Autodesk Inventor part; units mm, degrees
ref_plane "YZ Plane" through (0, 0, 0) normal (1, 0, 0) x (0, 1, 0)
ref_plane "XZ Plane" through (0, 0, 0) normal (0, 1, 0) x (-1, 0, 0)
ref_plane "XY Plane" through (0, 0, 0) normal (0, 0, 1) x (1, 0, 0)
sketch "Sketch1" plane through (0, 0, 0) normal (0, 1, 0) x (-1, 0, 0)
  circle A0 centre (0, 0) radius 1.4
  dimension "d0" = 2.8
extrude "Extrusion1" add sketch "Sketch1" along normal blind 5.5
sketch "Sketch2" plane through (0, 5.5, 0) normal (0, 1, 0) x (1, 0, 0)
  circle A0 centre (0, 0) radius 1.75
  line L0 (0, 0) -> (-1, 0)
  line L1 (-1, 0) -> (-0.5, 0.866)
  line L2 (-0.5, 0.866) -> (0.5, 0.866)
  line L3 (0.5, 0.866) -> (1, 0)
  line L4 (1, 0) -> (0.5, -0.866)
  line L5 (0.5, -0.866) -> (-0.5, -0.866)
  line L6 (-0.5, -0.866) -> (-1, 0)
  dimension "d3" = 3.5
  dimension "d4" = 1
extrude "Extrusion2" add sketch "Sketch2" along normal blind 1
thread "Thread1"
properties part number "Connector_3" material "Steel, Mild"
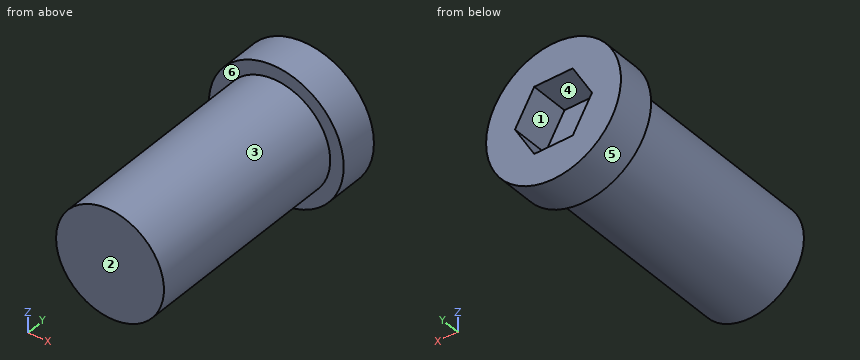
Read the model definition and answer for the solid it produces. Units are mm, in the model's axes. Face numbers are marked on the shaded views. A direction names the side the tool comes from. Give positions to 0.01 mm unless a question says otherwise; leave off trailing zeros. Loops run counter-clockwise (first coordinate to the right, second up) from the corner with the lowest first, then second, coordinate; pieces in that order, holes last. Notation, with made-up numbers: (12.5, 43) -> (25.5, 43) arc R22 cw to (25.5, 76) -> close; hole circle Ø6 at (83, 50.5). An arc over 180 degrees is marked (long way). Use a Markdown table: item, result.
Q1. This flat-tipped pin is pushed along its axis until it touches: pin 1 (0.5 mm diameter, centred on x = 0.5, z = 0, fed in from +Y). Where does it stop, or does it pass through?
Solved:
| item | result |
|---|---|
| pin 1 | stops at y = 5.5 |
Q2. Find the intervals of material crossed by line 1 along Z through (x, y) = (-0.05, 6); line 2 along Y through (x, z) = (-0.05, -0.15); line 3 along Y through (x, z) = (-1.55, 0.5), in increasing order.
Solved:
| item | result |
|---|---|
| line 1 | z = -1.75 to -0.87, 0.87 to 1.75 |
| line 2 | y = 0 to 5.5 |
| line 3 | y = 5.5 to 6.5 |
Q3. Section A-A, the plane x = 0 is taken. Determine the outline of the cut face in (y, z).
Solved:
| item | result |
|---|---|
| outline | (0, -1.4) -> (5.5, -1.4) -> (5.5, -1.75) -> (6.5, -1.75) -> (6.5, -0.87) -> (5.5, -0.87) -> (5.5, 0.87) -> (6.5, 0.87) -> (6.5, 1.75) -> (5.5, 1.75) -> (5.5, 1.4) -> (0, 1.4) -> close |
Q4. Section C-C, the plane z = 0.75 is taken. Determine the outline of the cut face in (x, y), then the cut area to 3 significant figures.
Solved:
| item | result |
|---|---|
| outline | (-1.58, 5.5) -> (-1.18, 5.5) -> (-1.18, 0) -> (1.18, 0) -> (1.18, 5.5) -> (1.58, 5.5) -> (1.58, 6.5) -> (0.57, 6.5) -> (0.57, 5.5) -> (-0.57, 5.5) -> (-0.57, 6.5) -> (-1.58, 6.5) -> close |
| area | 15.0 mm^2 |
Q5. Determine the mould class of the marked faces 4, 5 and 6 for opening direction Z: pulls with the +Z half, pulls with the -Z half, needs draft (parallel to the pull), parting line crosses it, or undercut.
Solved:
| item | result |
|---|---|
| face 4 | undercut |
| face 5 | parting line crosses it |
| face 6 | needs draft |
Q6. Section B-B, the plane y = 4.75 is taken. Determine the outline of the cut face in (x, z).
Solved:
| item | result |
|---|---|
| outline | circle Ø2.8 at (0, 0) |
Q7. Section D-D, the plane z = -0.95 is taken. Determine the outline of the cut face in (x, y), then the cut area to 3 significant figures.
Solved:
| item | result |
|---|---|
| outline | (-1.47, 5.5) -> (-1.03, 5.5) -> (-1.03, 0) -> (1.03, 0) -> (1.03, 5.5) -> (1.47, 5.5) -> (1.47, 6.5) -> (-1.47, 6.5) -> close |
| area | 14.3 mm^2 |
Q8. A tool of negligible diameter and unlimited length cuts with its end or side. For the marked faces 1, 2 and 3, from which of +Z, -Z, +X, -X, +Y, -Y can it reach the whole face along a straight path? Write none if from no direction.
Solved:
| item | result |
|---|---|
| face 1 | +Y |
| face 2 | +Z, -Z, +X, -X, -Y |
| face 3 | -Y |
